Autodesk Fusion 360 part; units mm, degrees
sketch "Sketch1" plane through (0, 0, 0) normal (0, 1, 0) x (1, 0, 0)
  circle A0 centre (0, 0) radius 2.1
  line L0 (-6.56, 5.4993) -> (-8.2, 5.4993)
  line L1 (-8.2, 5.4993) -> (-8.2, 3.1)
  line L2 (-8.2, 3.1) -> (-10, 4.9)
  line L3 (-10, 4.9) -> (-10, 10)
  line L4 (-10, 10) -> (-4.9, 10)
  line L5 (-4.9, 10) -> (-3.1, 8.2)
  line L6 (-3.1, 8.2) -> (-5.4993, 8.2)
  line L7 (-5.4993, 8.2) -> (-5.4993, 6.56)
  line L8 (-5.4993, 6.56) -> (-1.7793, 2.84)
  line L9 (-6.56, 5.4993) -> (-2.84, 1.7793)
  line L10 (0, 0) -> (-10, 10) construction
  line L11 (0, 0) -> (0, 5) construction
  line L12 (0, 0) -> (-5, 0) construction
  line L13 (-2.84, 1.7793) -> (-2.84, 0)
  line L14 (-1.7793, 2.84) -> (0, 2.84)
  line L15 (-8.2, -3.1) -> (-10, -4.9)
  line L16 (-6.56, -5.4993) -> (-8.2, -5.4993)
  line L17 (-10, -4.9) -> (-10, -10)
  line L18 (-4.9, -10) -> (-3.1, -8.2)
  line L19 (-5.4993, -6.56) -> (-1.7793, -2.84)
  line L20 (-6.56, -5.4993) -> (-2.84, -1.7793)
  line L21 (-1.7793, -2.84) -> (0, -2.84)
  line L22 (-3.1, -8.2) -> (-5.4993, -8.2)
  line L23 (-8.2, -5.4993) -> (-8.2, -3.1)
  line L24 (-10, -10) -> (-4.9, -10)
  line L25 (-5.4993, -8.2) -> (-5.4993, -6.56)
  line L26 (-2.84, -1.7793) -> (-2.84, 0)
  line L27 (4.9, 10) -> (3.1, 8.2)
  line L28 (2.84, -1.7793) -> (2.84, 0)
  line L29 (6.56, -5.4993) -> (2.84, -1.7793)
  line L30 (1.7793, 2.84) -> (0, 2.84)
  line L31 (5.4993, -8.2) -> (5.4993, -6.56)
  line L32 (5.4993, -6.56) -> (1.7793, -2.84)
  line L33 (10, 10) -> (4.9, 10)
  line L34 (2.84, 1.7793) -> (2.84, 0)
  line L35 (3.1, 8.2) -> (5.4993, 8.2)
  line L36 (10, -10) -> (4.9, -10)
  line L37 (1.7793, -2.84) -> (0, -2.84)
  line L38 (5.4993, 6.56) -> (1.7793, 2.84)
  line L39 (4.9, -10) -> (3.1, -8.2)
  line L40 (6.56, 5.4993) -> (2.84, 1.7793)
  line L41 (5.4993, 8.2) -> (5.4993, 6.56)
  line L42 (3.1, -8.2) -> (5.4993, -8.2)
  line L43 (10, -4.9) -> (10, 4.9) construction
  line L44 (20, 0) -> (30, 10) construction
  line L45 (26.56, -5.4993) -> (28.2, -5.4993)
  line L46 (23.1, 8.2) -> (25.4993, 8.2)
  line L47 (30, 4.9) -> (30, 10)
  line L48 (26.56, 5.4993) -> (22.84, 1.7793)
  line L49 (22.84, -1.7793) -> (22.84, 0)
  line L50 (30, -4.9) -> (30, -10)
  line L51 (25.4993, -8.2) -> (25.4993, -6.56)
  line L52 (23.1, -8.2) -> (25.4993, -8.2)
  line L53 (28.2, 5.4993) -> (28.2, 3.1)
  line L54 (28.2, 3.1) -> (30, 4.9)
  line L55 (20, 0) -> (20, 5) construction
  line L56 (20, 0) -> (25, 0) construction
  line L57 (30, -10) -> (24.9, -10)
  line L58 (26.56, -5.4993) -> (22.84, -1.7793)
  line L59 (24.9, -10) -> (23.1, -8.2)
  line L60 (25.4993, 8.2) -> (25.4993, 6.56)
  line L61 (28.2, -3.1) -> (30, -4.9)
  line L62 (22.84, 1.7793) -> (22.84, 0)
  line L63 (28.2, -5.4993) -> (28.2, -3.1)
  line L64 (10, -10) -> (15.1, -10)
  line L65 (16.9, 8.2) -> (14.5007, 8.2)
  line L66 (18.2207, 2.84) -> (20, 2.84)
  line L67 (14.5007, -6.56) -> (18.2207, -2.84)
  line L68 (15.1, 10) -> (16.9, 8.2)
  line L69 (13.44, 5.4993) -> (17.16, 1.7793)
  line L70 (18.2207, -2.84) -> (20, -2.84)
  line L71 (17.16, 1.7793) -> (17.16, 0)
  line L72 (15.1, -10) -> (16.9, -8.2)
  line L73 (14.5007, 6.56) -> (18.2207, 2.84)
  line L74 (17.16, -1.7793) -> (17.16, 0)
  line L75 (21.7793, 2.84) -> (20, 2.84)
  line L76 (30, 10) -> (24.9, 10)
  line L77 (26.56, 5.4993) -> (28.2, 5.4993)
  line L78 (24.9, 10) -> (23.1, 8.2)
  line L79 (25.4993, -6.56) -> (21.7793, -2.84)
  line L80 (14.5007, 8.2) -> (14.5007, 6.56)
  line L81 (10, 10) -> (15.1, 10)
  circle A1 centre (20, 0) radius 2.1
  line L82 (14.5007, -8.2) -> (14.5007, -6.56)
  line L83 (21.7793, -2.84) -> (20, -2.84)
  line L84 (16.9, -8.2) -> (14.5007, -8.2)
  line L85 (25.4993, 6.56) -> (21.7793, 2.84)
  line L86 (13.44, -5.4993) -> (17.16, -1.7793)
  line L87 (6.56, 5.4993) -> (7.2993, 6.2387)
  line L88 (7.2993, 6.2387) -> (7.2993, 8.2)
  line L89 (7.2993, 8.2) -> (12.7007, 8.2)
  line L90 (12.7007, 8.2) -> (12.7007, 6.2387)
  line L91 (12.7007, 6.2387) -> (13.44, 5.4993)
  line L92 (6.56, -5.4993) -> (7.2993, -6.2387)
  line L93 (7.2993, -6.2387) -> (7.2993, -8.2)
  line L94 (7.2993, -8.2) -> (12.7007, -8.2)
  line L95 (12.7007, -8.2) -> (12.7007, -6.2387)
  line L96 (12.7007, -6.2387) -> (13.44, -5.4993)
  point P0 (5, 0)
  point P1 (15, 0)
  point P2 (20, 0)
  point P3 (20, 0)
  dimension "d1" = 4.2
  dimension "d2" = 10
  dimension "d3" = 10
  dimension "d4" = 3.1
  dimension "d5" = 1.8
  dimension "d6" = 0
  dimension "d7" = 1.5
  dimension "d8" = 1.64
  dimension "d9" = 135
  dimension "d10" = 0
  dimension "d11" = 2.84
  dimension "d12" = 0
  dimension "d13" = 0
  dimension "d14" = 20
  dimension "d15" = 0
  dimension "d16" = 0
extrude "Extrude1" add sketch "Sketch1" along normal mid plane 460
equation "d4 = ( 6.2 / 2 ) * 1 mm"
equation "d6 = d10"
equation "d10 = d9"
equation "d11 = ( 5.68 / 2 ) * 1 mm"
equation "d12 = d19"
equation "d13 = d13"
equation "d15 = d10"
equation "d16 = d29"
Could you check a few things on this model? Use its own coordinates, in mm. Give positions to 0.01 mm unless a question says otherwise; leave off trailing zeros.
Item 1: If we section it at A-A, the plane y = -199: Count the separate pieces of the cut face and the enclosed holes in it, plus the area to 3 significant figures.
Item 2: I need wall thicknesses on line 1 (X direction, y = -26.5, z = 0); line 2 (Z direction, x = 0, y = 87.5); line 3 (Z direction, x = 8.5, y = 73.5). Which ranges of each line are inside material? Lowest first, please.
Item 3: I'm going to push flat-ended pins straight in: pin 1 (1.2 mm diameter, centred on x = -4, y = 102, fed in from -Z); pin 2 (0.7 mm diameter, centred on y = -1.5, z = -4.5, fed in from +X); pin 3 (1 mm diameter, centred on x = 18, y = 33.5, fed in from +Z). Where does each tip first touch, or does it pass through?
Values:
1. separate pieces: 1
1. enclosed holes: 3
1. area: 255 mm2
2. line 1: x = -2.84 to -2.1, 2.1 to 2.84, 17.16 to 17.9, 22.1 to 22.84
2. line 2: z = -2.84 to -2.1, 2.1 to 2.84
2. line 3: z = -10 to -8.2, 8.2 to 10
3. pin 1: stops at z = -9.7
3. pin 2: stops at x = 29.95
3. pin 3: stops at z = 3.56
